from build123d import *

# Parameters (mm, degrees)
SKETCH1_W           = 7
SKETCH1_H           = 7
SKETCH1_R           = 1.6
BOSS_EXTRUDE1_DEPTH = 5
SKETCH2_R           = 1.6
CUT_EXTRUDE1_DEPTH  = 10.287087811


with BuildPart() as part:
    # Sketch1 → Boss-Extrude1 (new, symmetric)
    with BuildSketch(Plane.XY):
        Rectangle(SKETCH1_W, SKETCH1_H)
        Circle(SKETCH1_R, mode=Mode.SUBTRACT)
    extrude(amount=BOSS_EXTRUDE1_DEPTH, both=True)

    # Sketch2 → Cut-Extrude1 (cut, through all)
    with BuildSketch(Plane(origin=(0, 3.5, 0), x_dir=(1, 0, 0), z_dir=(0, 1, 0))):
        with Locations((3.5, 0)):
            Circle(SKETCH2_R)
    extrude(amount=-CUT_EXTRUDE1_DEPTH, mode=Mode.SUBTRACT)


solid = part.part
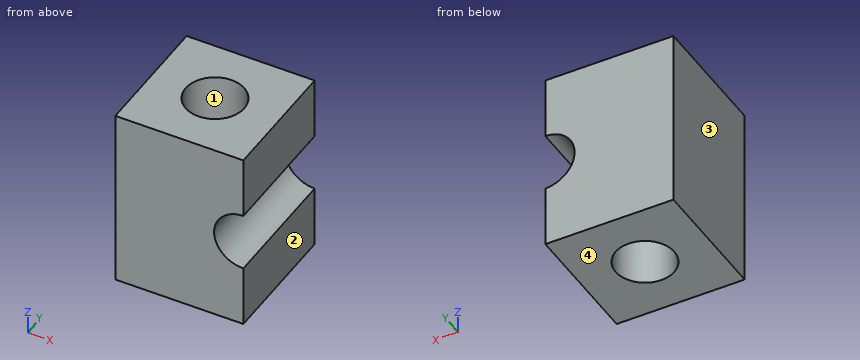
Check sheet for the modelled part. Datum: model origin and axes. Units: mm. Face numbers are marked on the shaded views. Coordinates: 2 decimals unless noted, no trailing zeros. Write each loop counter-clockwise with the first axis right and the second up, starting at its lowest first coordinate (ties: lowest second). Pieces come first, ordered by that corner, then holes.
Item 1: Scan lines: probe 1 along Y at (x, z) = (0, -0.25); probe 2 along Z at (x, y) = (3, -1.5); probe 3 along X at (y, z) = (-0.5, 2.75). Record each from-to range of solid material in increasing order.
Numbers:
probe 1: y = -3.5 to -1.6, 1.6 to 3.5
probe 2: z = -5 to -1.52, 1.52 to 5
probe 3: x = -3.5 to -1.52, 1.52 to 3.5
Item 2: Cross-section at D-D on y = -2.25. Record the boundary of the cut face in (x, z).
Numbers:
outline: (-3.5, -5) - (3.5, -5) - (3.5, -1.6) arc R1.6 cw to (3.5, 1.6) - (3.5, 5) - (-3.5, 5) - close
Item 3: Cross-section at A-A on y = 0. Record the boundary of the cut face in (x, z), then the cut area to 3 significant figures.
Numbers:
outline: (-3.5, -5) - (-1.6, -5) - (-1.6, 5) - (-3.5, 5) - close; (1.6, -5) - (3.5, -5) - (3.5, -1.6) arc R1.6 cw to (3.5, 1.6) - (3.5, 5) - (1.6, 5) - close
area: 34.0 mm2
Item 4: Mould release check, pull along X, two halves, no side actions. Record for the marked faces 1, 2, 3 and 4: released by +X, released by -X, zero draft, split by the parting line, or undercut.
Numbers:
face 1: undercut
face 2: released by +X
face 3: released by -X
face 4: zero draft
Item 5: Cross-section at B-B on x = 0. Record the boundary of the cut face in (y, z), then the cut area to 3 significant figures.
Numbers:
outline: (-3.5, -5) - (-1.6, -5) - (-1.6, 5) - (-3.5, 5) - close; (1.6, -5) - (3.5, -5) - (3.5, 5) - (1.6, 5) - close
area: 38.0 mm2
Item 6: Cross-section at C-C on z = -3.5. Record the boundary of the cut face in (x, y).
Numbers:
outline: (-3.5, -3.5) - (3.5, -3.5) - (3.5, 3.5) - (-3.5, 3.5) - close; hole circle Ø3.2 at (0, 0)
